from build123d import *

# Parameters (mm, degrees)
SKETCH1_R           = 15
BOSS_EXTRUDE2_DEPTH = 25
CUT_EXTRUDE1_DEPTH  = 10
SKETCH4_R           = 15
CUT_EXTRUDE2_DEPTH  = 15
CHAMFER1_SIZE       = 1
CHAMFER3_SIZE       = 1
CUT_EXTRUDE4_DEPTH  = 10
CUT_EXTRUDE5_DEPTH  = 1
CHAMFER5_SIZE       = 1


with BuildPart() as part:
    # Sketch1 → Boss-Extrude2 (new, symmetric)
    with BuildSketch(Plane(origin=(0, 0, 0), x_dir=(1, 0, 0), z_dir=(0, 1, 0))):
        with Locations(Location((0, 0, 0), (0, 0, 270))):
            Circle(SKETCH1_R)
    extrude(amount=BOSS_EXTRUDE2_DEPTH, both=True)

    # Sketch2 → Cut-Revolve1 (revolve, cut)
    with BuildSketch(Plane(origin=(0, 0, 0), x_dir=(0, 0, -1), z_dir=(1, 0, 0))):
        with BuildLine():
            Line((0, -9.125), (0, -25))
            Line((0, -25), (9.742785793, -25))
            ThreePointArc((9.742785793, -25), (10.709672947, -15.930380229), (4.636809248, -9.125))
            Line((4.636809248, -9.125), (0, -9.125))
        make_face()
    revolve(axis=Axis((0, -9.125, 0), (0, -1, 0)), mode=Mode.SUBTRACT)

    # Sketch3 → Cut-Extrude1 (cut)
    with BuildSketch(Plane(origin=(0, -25, 0), x_dir=(-1, 0, 0), z_dir=(0, -1, 0))):
        Polygon((19.052558883, 11), (18.552558883, 11.866025404), (9.892304845, 6.866025404), (0, 1.154700538), (-9.892304845, 6.866025404), (-18.552558883, 11.866025404), (-19.052558883, 11), (-19.552558883, 10.133974596), (-10.892304845, 5.133974596), (-1, -0.577350269), (-1, -12), (-1, -22), (0, -22), (1, -22), (1, -12), (1, -0.577350269), (10.892304845, 5.133974596), (19.552558883, 10.133974596), align=None)
    extrude(amount=-CUT_EXTRUDE1_DEPTH, mode=Mode.SUBTRACT)

    # Sketch4 → Cut-Extrude2 (cut)
    with BuildSketch(Plane(origin=(0, 25, 0), x_dir=(1, 0, 0), z_dir=(0, 1, 0))):
        with Locations(Location((0, 0, 0), (0, 0, 270))):
            Circle(SKETCH4_R)
    extrude(amount=-CUT_EXTRUDE2_DEPTH, mode=Mode.SUBTRACT)

    # Chamfer1
    chamfer1_edges = [part.edges().sort_by_distance(p)[0] for p in [
        (0, -25, -15),
        (-12.990381057, -25, 7.5),
        (12.990381057, -25, 7.5),
    ]]
    chamfer(chamfer1_edges, length=CHAMFER1_SIZE)

    # Chamfer3
    chamfer3_edges = [part.edges().sort_by_distance(p)[0] for p in [
        (12.990381057, -15, -7.5),
        (0.500278319, -15, 14.991655066),
        (-12.990381057, -15, -7.5),
    ]]
    chamfer(chamfer3_edges, length=CHAMFER3_SIZE)

    # Chamfer4: read off the stored shape, not the designer's step
    # Chamfer4 outline → Chamfer4 (revolve, cut)
    with BuildSketch(Plane.XY):
        Polygon((10.907310457, -25), (10.212304822, -24.094251023), (0, -24.094251023), (0, -25), align=None)
    revolve(axis=Axis((0, 0, 0), (0, 1, 0)), mode=Mode.SUBTRACT)

    # Sketch5 → Cut-Extrude4 (cut)
    with BuildSketch(Plane(origin=(0, 10, 0), x_dir=(1, 0, 0), z_dir=(0, 1, 0))):
        with BuildLine():
            Line((-5.099019514, -5.5), (5.099019514, -5.5))
            ThreePointArc((5.099019514, -5.5), (0, 7.5), (-5.099019514, -5.5))
        make_face()
    extrude(amount=-CUT_EXTRUDE4_DEPTH, mode=Mode.SUBTRACT)

    # Sketch7 → Cut-Extrude5 (cut, symmetric)
    with BuildSketch(Plane(origin=(0, 3.75, 0), x_dir=(1, 0, 0), z_dir=(0, 1, 0))):
        with BuildLine():
            Line((-5.477225575, -6.5), (5.477225575, -6.5))
            ThreePointArc((5.477225575, -6.5), (0, 8.5), (-5.477225575, -6.5))
        make_face()
    extrude(amount=CUT_EXTRUDE5_DEPTH, both=True, mode=Mode.SUBTRACT)

    # Chamfer5
    chamfer5_edges = [part.edges().sort_by_distance(p)[0] for p in [
        (0, 10, -7.5),
        (0, 10, 5.5),
        (0, 10, -15),
    ]]
    chamfer(chamfer5_edges, length=CHAMFER5_SIZE)


solid = part.part
Can you work these out from the model? Positions are in its coordinate system, mm. A direction names the side the tool comes from. Coordinates: 2 decimals unless noted, no trailing zeros. Write each loop counter-clockwise with the first axis right and the second up, starting at its lowest first coordinate (ties: lowest second). Pieces come first, ordered by that corner, then holes.
Q1. Imagine slicing it at D-D, the plane y = -10.5. List the corners of the cut face in (x, z) for me, plus the area to 3 significant figures.
Results found:
outline: circle Ø30 at (0, 0); hole circle Ø13.83 at (0, 0)
area: 557 mm2
Q2. Imagine slicing it at A-A, the plane y = -19.5. List the corners of the cut face in (x, z) for me, plus the area to 3 significant figures.
Results found:
outline: (-13.46, -6.62) - (-10.2, -4.74) arc R11.25 cw to (-1, 11.2) - (-1, 14.97) arc R15 ccw to start; (-12.46, -8.35) arc R15 ccw to (12.46, -8.35) - (9.2, -6.47) arc R11.25 cw to (-9.2, -6.47) - close; (1, 11.2) arc R11.25 cw to (10.2, -4.74) - (13.46, -6.62) arc R15 ccw to (1, 14.97) - close
area: 287 mm2
Q3. Imagine slicing it at B-B, the plane z = 0. List the corners of the cut face in (x, y) for me (3 decimals), plus the area to 3 significant figures.
Results found:
outline: (-15, -24) - (-14, -25) - (-10.907, -25) - (-10.212, -24.094) arc R11.25 cw to (-4.637, -9.125) - (4.637, -9.125) arc R11.25 cw to (10.212, -24.094) - (10.907, -25) - (14, -25) - (15, -24) - (15, 9) - (14, 10) - (8.5, 10) - (7.5, 9) - (7.5, 4.75) - (8.5, 4.75) - (8.5, 2.75) - (7.5, 2.75) - (7.5, 0) - (-7.5, 0) - (-7.5, 2.75) - (-8.5, 2.75) - (-8.5, 4.75) - (-7.5, 4.75) - (-7.5, 9) - (-8.5, 10) - (-14, 10) - (-15, 9) - close
area: 578 mm2
Q4. If we mould it in two halves opening along X, with no side actions, what happens to faces 4 (the face through (0, 10, 9)), 5 (the face through (0.66, -7.269, -14.985)), 6 (the face through (0, 0, -1)), 7 (the face through (-12.54, -14.51, -7.26))? For each: +X half, -X half, draft (parallel to the pull), parting line (faces both ways), or undercut.
Results found:
face 4: draft
face 5: parting line
face 6: undercut
face 7: undercut
Q5. Imagine slicing it at C-C, the plane x = 0. List the corners of the cut face in (y, z) for me (3 decimals).
Results found:
outline: (-25, -14) - (-24, -15) - (9, -15) - (10, -14) - (10, -8.5) - (9, -7.5) - (4.75, -7.5) - (4.75, -8.5) - (2.75, -8.5) - (2.75, -7.5) - (0, -7.5) - (0, 5.5) - (2.75, 5.5) - (2.75, 6.5) - (4.75, 6.5) - (4.75, 5.5) - (9, 5.5) - (10, 6.5) - (10, 14) - (9, 15) - (-14, 15) - (-15, 14) - (-15, 10.364) arc R11.25 cw to (-9.125, 4.637) - (-9.125, -4.637) arc R11.25 cw to (-24.094, -10.212) - (-25, -10.907) - close
Q6. Which directions (+Z, -Z, +X, -X, +Y, -Y) give clear straight access to the entire face, cutting with the end or side of a thin tool? Please do faces 1 (the face through (0.251, 6.905, -7.496)), 2 (the face through (0, -15, 12)), 3 (the face through (8.87, -24.24, 5.28)).
Results found:
face 1: +Y
face 2: +Z, -Y
face 3: -Y
Q7. For P1, Ø1.3, axis at x = -1, y = 6.5, coming from the -Z side; P2, Ø4, axis at x = -2, z = 2, coming from the +Y side; P3, Ø1, axis at x = 5, y = -3.5, coming from the -Z side, each with a flat end and sliding along its axis, tell me the tip position at first contact or that it passes through.
Results found:
P1: stops at z = -15
P2: stops at y = 0
P3: stops at z = -14.31
Q8. Please list where these lines run through material, in increasing order: L1, parallel to X at y = 0.6, z = 0; L2, parallel to X at y = 3.5, z = 0; L3, parallel to Z at x = 0.25, y = 6.5.
Results found:
L1: x = -15 to -7.5, 7.5 to 15
L2: x = -15 to -8.5, 8.5 to 15
L3: z = -15 to -7.5, 5.5 to 15
